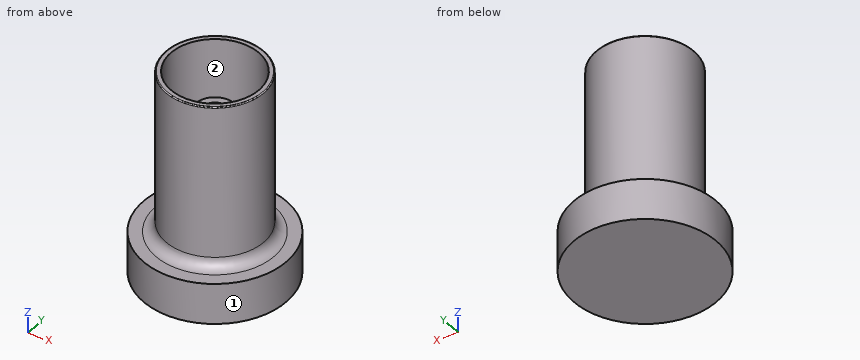
```python
from build123d import *

# Parameters (mm, degrees)
SKETCH1_R           = 7
BOSS_EXTRUDE1_DEPTH = 4
SKETCH2_R           = 4.791287292
BOSS_EXTRUDE2_DEPTH = 16
SKETCH3_R           = 4.310359808
CUT_EXTRUDE1_DEPTH  = 16
SKETCH4_R           = 1.889075337
SKETCH4_R_2         = 1.191130081
BOSS_EXTRUDE3_DEPTH = 12
FILLET1_R           = 1
FILLET2_R           = 0.1


with BuildPart() as part:
    # Sketch1 → Boss-Extrude1 (new body)
    with BuildSketch(Plane.XY):
        Circle(SKETCH1_R)
    extrude(amount=BOSS_EXTRUDE1_DEPTH)

    # Sketch2 → Boss-Extrude2 (add)
    with BuildSketch(Plane.XY.offset(4)):
        Circle(SKETCH2_R)
    extrude(amount=BOSS_EXTRUDE2_DEPTH)

    # Sketch3 → Cut-Extrude1 (cut)
    with BuildSketch(Plane.XY.offset(20)):
        Circle(SKETCH3_R)
    extrude(amount=-CUT_EXTRUDE1_DEPTH, mode=Mode.SUBTRACT)

    # Sketch4 → Boss-Extrude3 (add)
    with BuildSketch(Plane.XY.offset(4)):
        Circle(SKETCH4_R)
        Circle(SKETCH4_R_2, mode=Mode.SUBTRACT)
    extrude(amount=BOSS_EXTRUDE3_DEPTH)

    # Fillet1
    fillet1_edges = [part.edges().sort_by_distance(p)[0] for p in [
        (-4.791287292, 0, 4),
    ]]
    fillet(fillet1_edges, radius=FILLET1_R)

    # Fillet2
    fillet2_edges = [part.edges().sort_by_distance(p)[0] for p in [
        (-4.791287292, 0, 20),
    ]]
    fillet(fillet2_edges, radius=FILLET2_R)


solid = part.part
```
Input: part model. Units: mm. Frame: model coordinates. Face numbers are marked on the shaded views. A direction names the side the tool comes from. Give positions to 0.01 mm unless a question says otherwise; leave off trailing zeros. Order: outer loops, then holes, each group sorted by start corner. A loop starts at its lowest first (then second) coordinate and runs counter-clockwise, first axis right, second up. Notation, with made-up numbers: M 65.25,0 L 90.25,0 A13 cw 90.25,22 Z; hole C -20.75,-39 d6. An arc over 180 degrees is marked long. Return JSON: item names as keys, results as strings.
1) Contact query for flat-ended pins moving along their axis: pin 1 (2.5 mm diameter, centred on x = 0, y = 0, fed in from +Z); pin 2 (0.7 mm diameter, centred on x = 0, y = 0.5, fed in from +Z); pin 3 (2 mm diameter, centred on x = 0.5, z = 15, fed in from -Y). Output: stop coordinate, or through.
Taken from the geometry:
{"pin 1": "stops at z = 16", "pin 2": "stops at z = 4", "pin 3": "stops at y = -4.79"}
2) Section query B-B on z = 9. Output: boundary loops of the cut face in (x, y).
Taken from the geometry:
{"outline": "C 0,0 d9.58; C 0,0 d3.78; hole C 0,0 d8.62; hole C 0,0 d2.38"}
3) Access query for the marked faces 1 and 2. Directions: +Z, -Z, +X, -X, +Y, -Y. A direction counts if a zero-diameter tool reaches every point of the face in a straight line with its end or side. Return the directions, or none.
Taken from the geometry:
{"face 1": "+Z, -Z", "face 2": "+Z"}
4) Section query A-A on y = 0. Output: boundary loops of the cut face in (x, z).
Taken from the geometry:
{"outline": "M -7,0 L 7,0 L 7,4 L 5.79,4 A1 cw 4.79,5 L 4.79,19.9 A0.1 ccw 4.69,20 L 4.31,20 L 4.31,4 L 1.89,4 L 1.89,16 L 1.19,16 L 1.19,4 L -1.19,4 L -1.19,16 L -1.89,16 L -1.89,4 L -4.31,4 L -4.31,20 L -4.69,20 A0.1 ccw -4.79,19.9 L -4.79,5 A1 cw -5.79,4 L -7,4 Z"}
5) Line query: L1, parallel to Y at x = 0, z = 14.25; L2, parallel to Y at x = 0, z = 16.75; L3, parallel to X at y = 2, z = 18.75. Output: solid intervals per line, ascending. Write a range as [from, to].
Taken from the geometry:
{"L1": "y = [-4.79, -4.31], [-1.89, -1.19], [1.19, 1.89], [4.31, 4.79]", "L2": "y = [-4.79, -4.31], [4.31, 4.79]", "L3": "x = [-4.35, -3.82], [3.82, 4.35]"}
